For this review, take the finished solid that the model builds, in its own axes (mm). A direction names the side the tool comes from. Give positions to 0.01 mm unless a question says otherwise; leave off trailing zeros. Order: outer loops, then holes, each group sorted by start corner. A loop starts at its lowest first (then second) coordinate and runs counter-clockwise, first axis right, second up. Notation, with made-up numbers: (82.25, -23.75) -> (107.25, -23.75) arc R16 cw to (107.25, 0.25) -> close; hole circle Ø9 at (-12.5, -13). An arc over 180 degrees is marked (long way). Return JSON: item names as keys, results as strings. Group by question number.
1) Add section C-C (z = -77.5). Give the boundary of the cut face in (x, y), then the cut area to 3 significant figures.
2) Add section A-A (z = -31). Give the boundary of the cut face in (x, y).
3) Insertion check: P1, Ø1.2, axis at x = -15, y = -15.5, coming from the +Z side; P2, Ø2, axis at x = 16, y = -15.5, coming from the +Z side; P3, Ø1, axis at x = -8.5, y = -3, coming from the +Z side; P4, Ø3, axis at y = -15.5, z = -55.5, coming from the +X side. Each pin has a flat end and moves straight along its axis. Give the tip position at first contact, or say it passes through.
4) To check wall thickness, follow line 1 along Y through (x, z) = (15.5, -28.5); line 2 along Z through (x, y) = (9, 1). State the ranges of each line that lie inside material, in increasing order.
5) For faces 4 (the face through (0, 2, -10)), 5 (the face through (9, -9, -24)), 6 (the face through (-17.88, -17.79, -53.7)), 7 (the face through (-19, 17, -32)), 8 (the face through (21.15, 0, -54)), list the 3-axis set-ups (+Z, -Z, +X, -X, +Y, -Y) from which the entire face can be reached by the end or side of a thin tool; tool diameter is ignored.
6) The part is to be moulded in two halves that separate along X. For faces 1 (the face through (-17.436, -17.525, -75.746)), 2 (the face through (-16, -15, -34)), 3 (the face through (17.79, -17.88, -53.7)), say which applies: released by +X, released by -X, zero draft, split by the parting line, or undercut.
from build123d import *

# Parameters (mm, degrees)
SKETCH1_R           = 2.5
BOSS_EXTRUDE1_DEPTH = 22
SKETCH2_R           = 11
BOSS_EXTRUDE2_DEPTH = 2
BOSS_EXTRUDE3_DEPTH = 8
BOSS_EXTRUDE6_DEPTH = 0.5
BOSS_EXTRUDE4_DEPTH = 43
BOSS_EXTRUDE7_DEPTH = 0.5
BOSS_EXTRUDE5_DEPTH = 8
CHAMFER1_SIZE       = 0.5
SKETCH8_W           = 6.467116259
SKETCH8_H           = 1.343520631
CUT_EXTRUDE1_DEPTH  = 20
SKETCH9_R           = 1.25
CUT_EXTRUDE2_DEPTH  = 10


with BuildPart() as part:
    # Sketch1 → Boss-Extrude1 (new body)
    with BuildSketch(Plane.XY):
        Circle(SKETCH1_R)
    extrude(amount=-BOSS_EXTRUDE1_DEPTH)

    # Sketch2 → Boss-Extrude2 (add)
    with BuildSketch(Plane(origin=(0, 0, -22), x_dir=(-1, 0, 0), z_dir=(0, 0, -1))):
        Circle(SKETCH2_R)
    extrude(amount=BOSS_EXTRUDE2_DEPTH)

    # Sketch3 → Boss-Extrude3 (add)
    with BuildSketch(Plane(origin=(0, 0, -24), x_dir=(-1, 0, 0), z_dir=(0, 0, -1))):
        with BuildLine():
            Line((15.5, -21.15), (-15.5, -21.15))
            ThreePointArc((-15.5, -21.15), (-18.541473782, -18.541473782), (-21.15, -15.5))
            Line((-21.15, -15.5), (-21.15, 15.5))
            ThreePointArc((-21.15, 15.5), (-18.541473782, 18.541473782), (-15.5, 21.15))
            Line((-15.5, 21.15), (15.5, 21.15))
            ThreePointArc((15.5, 21.15), (18.541473782, 18.541473782), (21.15, 15.5))
            Line((21.15, 15.5), (21.15, -15.5))
            ThreePointArc((21.15, -15.5), (18.541473782, -18.541473782), (15.5, -21.15))
        make_face()
    extrude(amount=BOSS_EXTRUDE3_DEPTH)

    # Sketch6 → Boss-Extrude6 (add)
    with BuildSketch(Plane(origin=(0, 0, -32), x_dir=(-1, 0, 0), z_dir=(0, 0, -1))):
        Polygon((-20.65, -14.31162722), (-14.31162722, -20.65), (14.31162722, -20.65), (20.65, -14.31162722), (20.65, 14.31162722), (14.31162722, 20.65), (-14.31162722, 20.65), (-20.65, 14.31162722), align=None)
    extrude(amount=BOSS_EXTRUDE6_DEPTH)

    # Sketch4 → Boss-Extrude4 (add)
    with BuildSketch(Plane(origin=(0, 0, -32.5), x_dir=(-1, 0, 0), z_dir=(0, 0, -1))):
        Polygon((-21.15, 14.518734001), (-14.518734001, 21.15), (14.518734001, 21.15), (21.15, 14.518734001), (21.15, -14.518734001), (14.518734001, -21.15), (-14.518734001, -21.15), (-21.15, -14.518734001), align=None)
    extrude(amount=BOSS_EXTRUDE4_DEPTH)

    # Sketch7 → Boss-Extrude7 (add)
    with BuildSketch(Plane(origin=(0, 0, -75.5), x_dir=(-1, 0, 0), z_dir=(0, 0, -1))):
        Polygon((-20.65, -14.31162722), (-14.31162722, -20.65), (14.31162722, -20.65), (20.65, -14.31162722), (20.65, 14.31162722), (14.31162722, 20.65), (-14.31162722, 20.65), (-20.65, 14.31162722), align=None)
    extrude(amount=BOSS_EXTRUDE7_DEPTH)

    # Sketch5 → Boss-Extrude5 (add)
    with BuildSketch(Plane(origin=(0, 0, -76), x_dir=(-1, 0, 0), z_dir=(0, 0, -1))):
        with BuildLine():
            Line((-15.5, -21.15), (15.5, -21.15))
            ThreePointArc((15.5, -21.15), (18.541473782, -18.541473782), (21.15, -15.5))
            Line((21.15, -15.5), (21.15, 15.5))
            ThreePointArc((21.15, 15.5), (18.541473782, 18.541473782), (15.5, 21.15))
            Line((15.5, 21.15), (-15.5, 21.15))
            ThreePointArc((-15.5, 21.15), (-18.541473782, 18.541473782), (-21.15, 15.5))
            Line((-21.15, 15.5), (-21.15, -15.5))
            ThreePointArc((-21.15, -15.5), (-18.541473782, -18.541473782), (-15.5, -21.15))
        make_face()
    extrude(amount=BOSS_EXTRUDE5_DEPTH)

    # Chamfer1
    chamfer1_edges = [part.edges().sort_by_distance(p)[0] for p in [
        (-2.5, 0, 0),
    ]]
    chamfer(chamfer1_edges, length=CHAMFER1_SIZE)

    # Sketch8 → Cut-Extrude1 (cut)
    with BuildSketch(Plane.XY):
        with Locations((0.298403281, 2.671760316)):
            Rectangle(SKETCH8_W, SKETCH8_H)
    extrude(amount=-CUT_EXTRUDE1_DEPTH, mode=Mode.SUBTRACT)

    # Sketch9 → Cut-Extrude2 (cut)
    with BuildSketch(Plane.XY.offset(-24)):
        with Locations((-15.5, 15.5)):
            Circle(SKETCH9_R)
        with Locations((15.5, 15.5)):
            Circle(SKETCH9_R)
        with Locations((15.5, -15.5)):
            Circle(SKETCH9_R)
        with Locations((-15.5, -15.5)):
            Circle(SKETCH9_R)
    extrude(amount=-CUT_EXTRUDE2_DEPTH, mode=Mode.SUBTRACT)


solid = part.part
Evaluation:
{
 "1": {"outline": "(-21.15, -15.5) arc R26.22 ccw to (-15.5, -21.15) -> (15.5, -21.15) arc R26.22 ccw to (21.15, -15.5) -> (21.15, 15.5) arc R26.22 ccw to (15.5, 21.15) -> (-15.5, 21.15) arc R26.22 ccw to (-21.15, 15.5) -> close", "area": "1,730 mm^2"},
 "2": {"outline": "(-21.15, -15.5) arc R26.22 ccw to (-15.5, -21.15) -> (15.5, -21.15) arc R26.22 ccw to (21.15, -15.5) -> (21.15, 15.5) arc R26.22 ccw to (15.5, 21.15) -> (-15.5, 21.15) arc R26.22 ccw to (-21.15, 15.5) -> close; hole circle Ø2.5 at (-15.5, -15.5); hole circle Ø2.5 at (-15.5, 15.5); hole circle Ø2.5 at (15.5, -15.5); hole circle Ø2.5 at (15.5, 15.5)"},
 "3": {"P1": "z = -34", "P2": "z = -24", "P3": "z = -22", "P4": "x = 21.15"},
 "4": {"line 1": "-21.15 to -16.75, -14.25 to 14.25, 16.75 to 21.15", "line 2": "-84 to -22"},
 "5": {"face 4": "+Z, +X, -X, +Y", "face 5": "+Z", "face 6": "-X, -Y", "face 7": "none", "face 8": "+Z, -Z, +X, +Y, -Y"},
 "6": {"face 1": "released by -X", "face 2": "undercut", "face 3": "released by +X"}
}
